Part model, mm, in its own coordinate system. A direction names the side the tool comes from. Round coordinates to 2 decimals unless told otherwise and drop trailing zeros. Loops run counter-clockwise (first coordinate to the right, second up) from the corner with the lowest first, then second, coordinate; pieces in that order, holes last.
Autodesk Inventor part; units mm, degrees
ref_plane "YZ Plane" through (0, 0, 0) normal (1, 0, 0) x (0, 1, 0)
ref_plane "XZ Plane" through (0, 0, 0) normal (0, 1, 0) x (-1, 0, 0)
ref_plane "XY Plane" through (0, 0, 0) normal (0, 0, 1) x (1, 0, 0)
sketch "Sketch1" plane through (0, 0, 0) normal (0, 1, 0) x (-1, 0, 0)
  line L0 (0, 0) -> (80, 0)
  line L1 (20, 5) -> (0, 5)
  line L2 (0, 5) -> (0, 0)
  line L3 (46.5184, 5) -> (46.5184, 80)
  circle A0 centre (26.5184, 80) radius 20
  line L4 (26.5184, 100) -> (-123.4816, 100)
  circle A1 centre (-123.4816, 80) radius 20
  line L5 (-123.4816, 60) -> (-39.7913, 60)
  arc A2 (20, 5) -> (-39.7913, 60) centre (-39.7913, 0) ccw
  line L6 (46.5184, 5) -> (66.5184, 5)
  line L7 (66.5184, 5) -> (66.5184, 0)
  line L8 (66.5184, 0) -> (46.5184, 0)
  point P0 (16.5184, 60)
  dimension "d1" = 75
  dimension "d2" = 40
  dimension "d3" = 150
  dimension "d4" = 140
  dimension "d7" = 40
  dimension "d10" = 5
  dimension "d11" = 5
extrude "Extrusion1" add sketch "Sketch1" along normal blind 50
sketch "Sketch2" plane through (-20, 0, 5) normal (0, 0, 1) x (1, 0, 0)
  circle A0 centre (10, 25) radius 3.5
  line L0 (20, 0) -> (20, 50)
  line L1 (0, 50) -> (20, 50)
  circle A1 centre (-36.5184, 25) radius 3.5
  line L2 (-46.5184, 0) -> (-46.5184, 50)
  line L3 (-46.5184, 50) -> (-26.5184, 50)
  dimension "d14" = 7
  dimension "d15" = 10
  dimension "d16" = 25
  dimension "d17" = 7
  dimension "d18" = 10
  dimension "d22" = 25
extrude "Extrusion2" cut sketch "Sketch2" against normal blind 20
sketch "Sketch3" plane through (0, 50, 0) normal (0, 1, 0) x (1, 0, 0)
  line L0 (-46.5184, -5) -> (-46.5184, -80)
  arc A0 (-20, -5) -> (39.7913, -60) centre (39.7913, 0) ccw
  line L1 (-26.5184, -100) -> (123.4816, -100)
  arc A1 (123.4816, -100) -> (123.4816, -60) centre (123.4816, -80) ccw
  line L2 (123.4816, -60) -> (39.7913, -60)
  arc A2 (-20, -5) -> (39.7913, -60) centre (39.7913, 0) ccw
  line L3 (-46.5184, -5) -> (-46.5184, -80)
  arc A3 (-46.5184, -80) -> (-26.5184, -100) centre (-26.5184, -80) ccw
  arc A4 (-46.5184, -80) -> (-26.5184, -100) centre (-26.5184, -80) ccw
  line L4 (-46.5184, -5) -> (-20, -5)
  line L5 (-26.5184, -97.5) -> (123.4816, -97.5)
  arc A5 (123.4816, -97.5) -> (123.4816, -62.5) centre (123.4816, -80) ccw
  line L6 (123.4816, -62.5) -> (39.7913, -62.5)
  arc A6 (-22.2571, -7.5) -> (39.7913, -62.5) centre (39.7913, 0) ccw
  line L7 (-22.2571, -7.5) -> (-44.0184, -7.5)
  line L8 (-44.0184, -7.5) -> (-44.0184, -80)
  line L9 (-26.5184, -97.5) -> (123.4816, -97.5)
  arc A7 (123.4816, -97.5) -> (123.4816, -62.5) centre (123.4816, -80) ccw
  line L10 (123.4816, -62.5) -> (39.7913, -62.5)
  arc A8 (-22.2571, -7.5) -> (39.7913, -62.5) centre (39.7913, 0) ccw
  line L11 (-22.2571, -7.5) -> (-44.0184, -7.5)
  line L12 (-44.0184, -7.5) -> (-44.0184, -80)
  arc A9 (-44.0184, -80) -> (-26.5184, -97.5) centre (-26.5184, -80) ccw
  point P0 (0, 0)
  point P1 (39.7913, -60)
  dimension "d24" = 2.5
  dimension "d25" = 2.5
extrude "Extrusion3" cut sketch "Sketch3" against normal blind 10 contours A9 L8 L7 A6 L6 A5 L5
sketch "Sketch4" plane through (0, 0, 0) normal (0, -1, 0) x (1, 0, 0)
  arc A0 (39.7913, 60) -> (-20, 5) centre (39.7913, 0) ccw
  line L0 (-20, 5) -> (-46.5184, 5)
  line L1 (-46.5184, 5) -> (-46.5184, 80)
  arc A1 (-26.5184, 100) -> (-46.5184, 80) centre (-26.5184, 80) ccw
  line L2 (123.4816, 60) -> (39.7913, 60)
  arc A2 (123.4816, 60) -> (123.4816, 100) centre (123.4816, 80) ccw
  line L3 (-26.5184, 100) -> (123.4816, 100)
  arc A3 (123.4816, 62.5) -> (123.4816, 97.5) centre (123.4816, 80) ccw
  line L4 (123.4816, 62.5) -> (39.7913, 62.5)
  arc A4 (39.7913, 62.5) -> (-22.2571, 7.5) centre (39.7913, 0) ccw
  line L5 (-22.2571, 7.5) -> (-44.0184, 7.5)
  line L6 (-44.0184, 7.5) -> (-44.0184, 80)
  arc A5 (-26.5184, 97.5) -> (-44.0184, 80) centre (-26.5184, 80) ccw
  line L7 (-26.5184, 97.5) -> (123.4816, 97.5)
  point P0 (0, 0)
  dimension "d28" = 2.5
extrude "Extrusion4" cut sketch "Sketch4" against normal blind 10 contours L4 A4 L5 L6 A5 L7 A3
properties part number "Pylon"
1) Slice it at A-A, the plane y = 25. Give the cut face in (x, z).
Values:
outline: (-66.52, 0) - (-60.02, 0) - (-60.02, 5) - (-66.52, 5) - close; (-53.02, 0) - (-13.5, 0) - (-13.5, 5) - (-20, 5) arc R60 cw to (39.79, 60) - (123.48, 60) arc R20 ccw to (123.48, 100) - (-26.52, 100) arc R20 ccw to (-46.52, 80) - (-46.52, 5) - (-53.02, 5) - close; (-6.5, 0) - (0, 0) - (0, 5) - (-6.5, 5) - close
2) Tool access for faces 4 (the face through (82, 5, 62.5)), 5 (the face through (-33, 45, 7.5)), 6 (the face through (82, 25, 60)), 7 (the face through (-0.367, 24.65, 44.579)): list every direction of +Z, -Z, +X, -X, +Y, -Y with a clear straight run to the whole face (end or side of a thin tool).
Values:
face 4: -Y
face 5: +Y
face 6: -Z, +X, +Y, -Y
face 7: +X, +Y, -Y
3) Slice it at D-D, the plane z = 29. Give the cut face in (x, y), then the cut area to 3 significant figures.
Values:
outline: (-46.52, 0) - (-44.02, 0) - (-44.02, 10) - (-15.57, 10) - (-15.57, 0) - (-12.73, 0) - (-12.73, 50) - (-15.57, 50) - (-15.57, 40) - (-44.02, 40) - (-44.02, 50) - (-46.52, 50) - close
area: 1,120 mm2
4) Drop flat-ended pins along their axis: pin 1 Ø5 at (x, y) = (-37, 5) entering from +Z; pin 2 Ø4 at (y, z) = (9, 17) entering from -X; pin 3 Ø5.5 at (y, z) = (21.5, 1.5) entering from +X. Give the stop position or say it passes through.
Values:
pin 1: stops at z = 98.34
pin 2: stops at x = -46.52
pin 3: stops at x = 0
5) Slice it at C-C, the plane x = 67.5. Give the cut face in (y, z).
Values:
outline: (0, 60) - (50, 60) - (50, 62.5) - (40, 62.5) - (40, 97.5) - (50, 97.5) - (50, 100) - (0, 100) - (0, 97.5) - (10, 97.5) - (10, 62.5) - (0, 62.5) - close
6) Wall check: line 1 along Y through (x, z) = (-10, 2.65); line 2 along Z through (x, y) = (80, 47.5); line 3 along Z through (x, y) = (-26.5, 45). Give the ranges that are in metal, low to high.
Values:
line 1: y = 0 to 21.5, 28.5 to 50
line 2: z = 60 to 62.5, 97.5 to 100
line 3: z = 0 to 7.5, 97.5 to 100
7) Mould opens along Z. For faces 1 (the face through (47, 5, 97.5)), 2 (the face through (143.477, 24.65, 79.56)), 3 (the face through (-66.518, 25, 3)) say: released by +Z, released by -Z, zero draft, split by the parting line, or undercut.
Values:
face 1: undercut
face 2: split by the parting line
face 3: zero draft
8) Slice it at B-B, the plane x = -10. Give the cut face in (y, z).
Values:
outline: (0, 0) - (21.5, 0) - (21.5, 5) - (0, 5) - close; (0, 33.48) - (50, 33.48) - (50, 37.78) - (40, 37.78) - (40, 97.5) - (50, 97.5) - (50, 100) - (0, 100) - (0, 97.5) - (10, 97.5) - (10, 37.78) - (0, 37.78) - close; (28.5, 0) - (50, 0) - (50, 5) - (28.5, 5) - close
